For this review, use the dimensioned drawing (mm, ordinates from the lowest corner) and the shaded views. Give positions to 0.01 mm unless a question says otherwise; leave off trailing zeros. Loops run counter-clockwise (first coordinate to the right, second up) from the corner with the lowest first, then second, coordinate; pieces in that order, holes last. Notation, with made-up numbers: (-14.75, -25.75) -> (36.25, -25.75) arc R23 ccw to (36.25, -8.75) -> close; hole circle Ø2 at (70, 1). An arc over 180 degrees is marked (long way). Write each question's results on one line, items separated by ' | '. Start each with the question number.
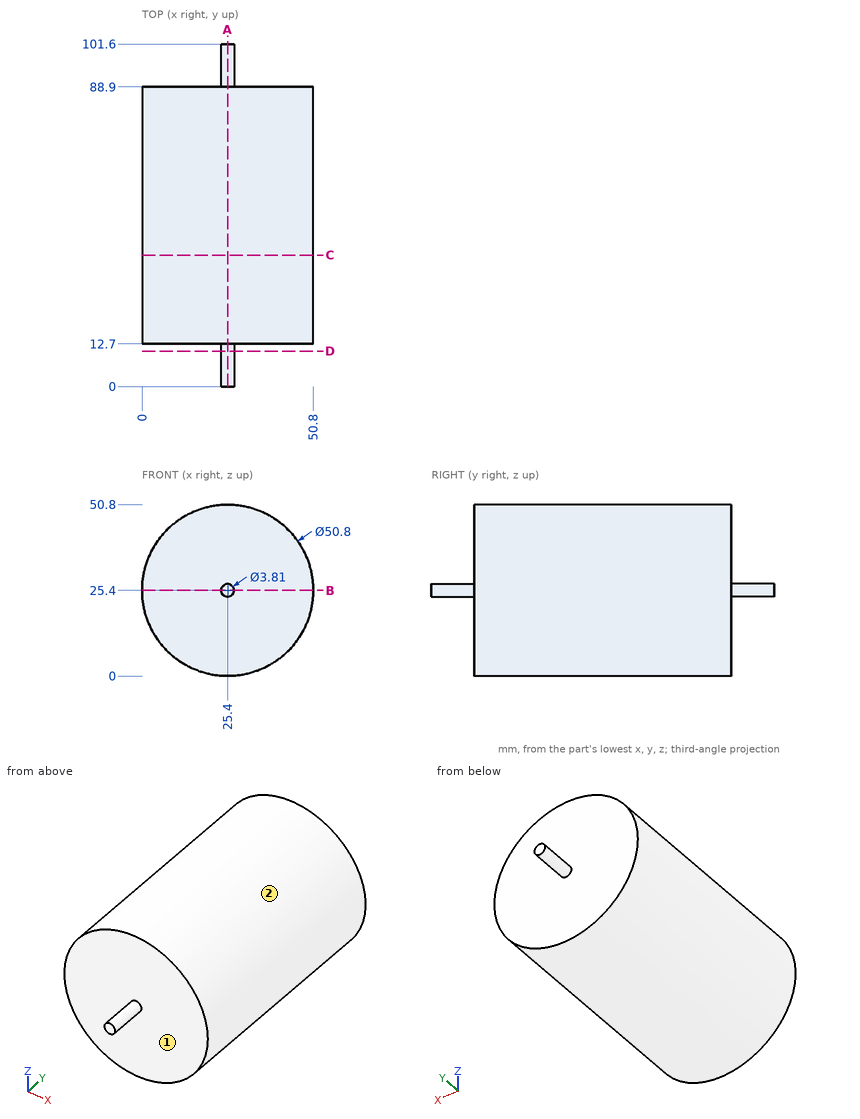
1. We need section B-B (z = 25.4). Write out the cut boundary in (x, y) (3 decimals), plus the area to 3 significant figures.
2. We need section A-A (x = 25.4). Write out the cut boundary in (y, z) (3 decimals).
3. For pin 1 Ø6 at (x, y) = (12.5, 90) entering from +Z; pin 2 Ø10 at (x, z) = (30.5, 9) entering from -Y; pin 3 Ø1 at (y, z) = (23, 42) entering from -X, all flat-tipped, find the tip position at first contact; note any pin that passes through.
4. Draft analysis for pull direction Z (two halves, no side actions). For the marked faces 1 and 2, state which applies: released by +Z, released by -Z, zero draft, split by the parting line, or undercut.
5. We need section C-C (y = 39). Write out the cut boundary in (x, z), plus the area to 3 significant figures.
6. We need section D-D (y = 10.5). Write out the cut boundary in (x, z) (3 decimals), plus the area to 3 significant figures.
7. Wall thickness on L1, parallel to X at y = 20, z = 26; L2, parallel to Y at x = 39, z = 30; L3, parallel to Z at x = 4.5, y = 17.5: over which ranges is each line inside the solid? List them lowest first.
Response:
1) outline: (0, 12.7) -> (23.495, 12.7) -> (23.495, 0) -> (27.305, 0) -> (27.305, 12.7) -> (50.8, 12.7) -> (50.8, 88.9) -> (27.305, 88.9) -> (27.305, 101.6) -> (23.495, 101.6) -> (23.495, 88.9) -> (0, 88.9) -> close | area: 3,970 mm2
2) outline: (0, 23.495) -> (12.7, 23.495) -> (12.7, 0) -> (88.9, 0) -> (88.9, 23.495) -> (101.6, 23.495) -> (101.6, 27.305) -> (88.9, 27.305) -> (88.9, 50.8) -> (12.7, 50.8) -> (12.7, 27.305) -> (0, 27.305) -> close
3) pin 1: stops at z = 48.7 | pin 2: stops at y = 12.7 | pin 3: stops at x = 5.75
4) face 1: zero draft | face 2: split by the parting line
5) outline: circle Ø50.8 at (25.4, 25.4) | area: 2,030 mm2
6) outline: circle Ø3.81 at (25.4, 25.4) | area: 11.4 mm2
7) L1: x = 0.01 to 50.79 | L2: y = 12.7 to 88.9 | L3: z = 10.97 to 39.83
